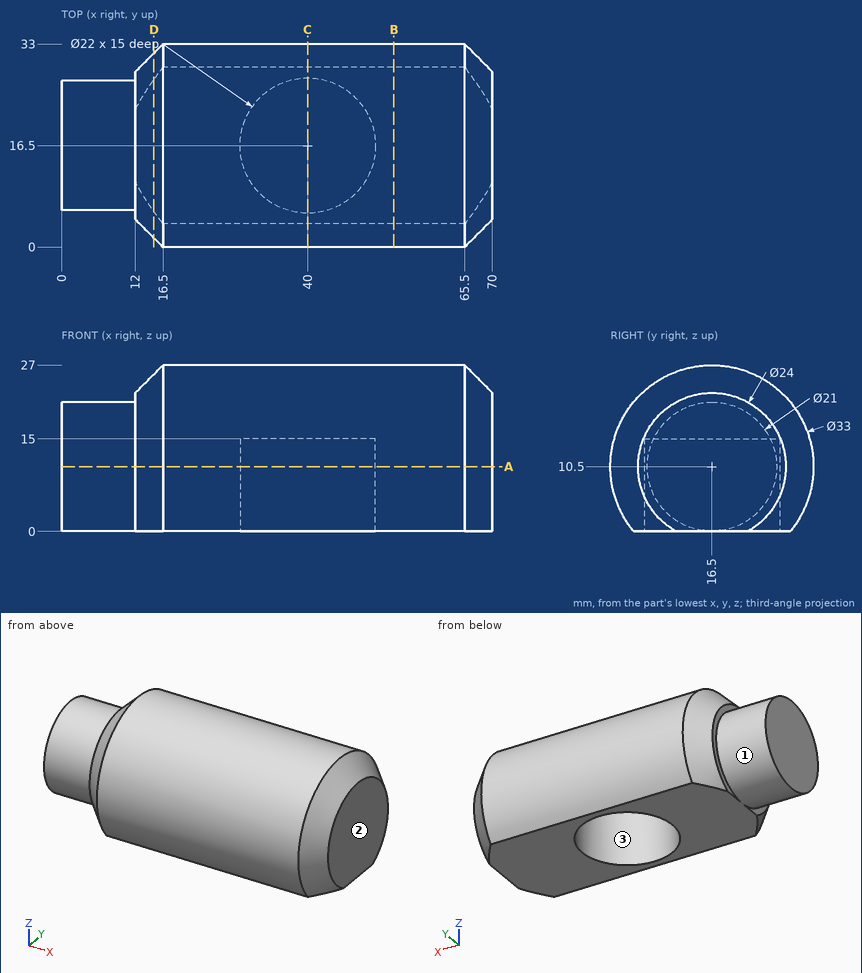
The drawing under review shows one solid part. Ordinate dimensions are in mm from its lowest x, y, z. Round coordinates to 2 decimals unless told otherwise and drop trailing zeros. Write each loop counter-clockwise with the first axis right and the second up, starting at its lowest first coordinate (ties: lowest second). Pieces come first, ordered by that corner, then holes. Notation, with made-up numbers: (-22.5, 81.25) -> (-4.5, 81.25) arc R26 ccw to (-4.5, 96.25) -> close; hole circle Ø11 at (-34, -22). An arc over 180 degrees is marked (long way). Put each result on its own line as item: value.
Q1. To check wall thickness, follow L1, parallel to Y at x = 40, z = 10.25; L2, parallel to X at y = 16.5, z = 11.5; L3, parallel to Y at x = 50, z = 4.75. State the ranges of each line that lie inside material, in increasing order. Write a range as [from, to].
Determined:
L1: y = [0, 5.5], [27.5, 33]
L2: x = [0, 29], [51, 70]
L3: y = [1.03, 11.92], [21.08, 31.97]
Q2. Consider section A-A on z = 10.5. State the section outline as (x, y) points.
Determined:
outline: (0, 6) -> (12, 6) -> (12, 4.5) -> (16.5, 0) -> (65.5, 0) -> (70, 4.5) -> (70, 28.5) -> (65.5, 33) -> (16.5, 33) -> (12, 28.5) -> (12, 27) -> (0, 27) -> close; hole circle Ø22 at (40, 16.5)
Q3. Clearance check with flat-ended pins moving along their axes: pin 1 Ø11 at (x, y) = (41, 14) entering from -Z; pin 2 Ø4 at (y, z) = (5, 24) entering from +X; pin 3 Ø4 at (x, z) = (58, 5.5) entering from -Y (3 decimals). State where each tip first meets the part, or that it passes through.
Determined:
pin 1: stops at z = 15
pin 2: stops at x = 66.27
pin 3: stops at y = 0.275
Q4. The part is to be moulded in two halves that separate along X. For the marked faces 1, 2 and 3, say which applies: released by +X, released by -X, zero draft, split by the parting line, or undercut.
Determined:
face 1: zero draft
face 2: released by +X
face 3: undercut
Q5. Consider section D-D on x = 15. State the section outline as (y, z) points.
Determined:
outline: (5.79, 0) -> (27.21, 0) arc R15 ccw (long way) to start
Q6. Consider section C-C on x = 40. State the section outline as (y, z) points.
Determined:
outline: (3.77, 0) -> (5.5, 0) -> (5.5, 15) -> (27.5, 15) -> (27.5, 0) -> (29.23, 0) arc R16.5 ccw (long way) to start
Q7. Consider section B-B on x = 54. State the section outline as (y, z) points, and give its area (3 significant figures).
Determined:
outline: (3.77, 0) -> (29.23, 0) arc R16.5 ccw (long way) to start
area: 749 mm^2
